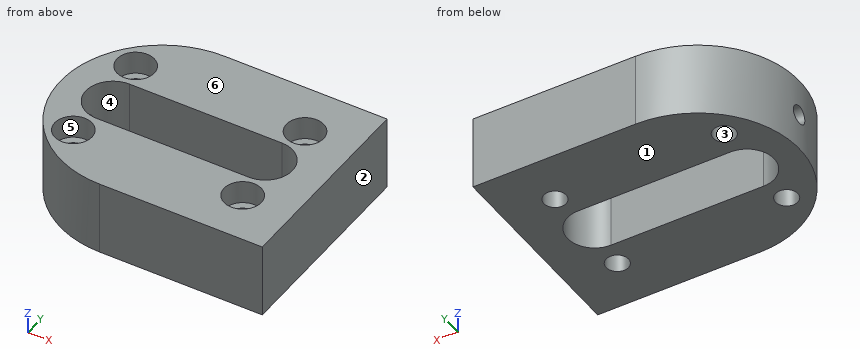
```python
from build123d import *

# Parameters (mm, degrees)
EXTRUDE_1_DEPTH           = 22
HOLE_WIZARD_1_D           = 6.6
HOLE_WIZARD_1_CBORE_D     = 11
HOLE_WIZARD_1_CBORE_DEPTH = 6.8
MM_1_REACH                = 86.291
MM_1_BORE_R               = 2.75


with BuildPart() as part:
    # 草图1 → 凸台-拉伸1 (new body)
    with BuildSketch(Plane.XY):
        with BuildLine():
            Line((-8, 30), (40, 30))
            Line((40, 30), (40, -30))
            Line((40, -30), (-8, -30))
            ThreePointArc((-8, -30), (-38, 0), (-8, 30))
        make_face()
        with BuildLine():
            Line((-22.5, 8), (22.5, 8))
            ThreePointArc((22.5, 8), (30.5, 0), (22.5, -8))
            Line((22.5, -8), (-22.5, -8))
            ThreePointArc((-22.5, -8), (-30.5, 0), (-22.5, 8))
        make_face(mode=Mode.SUBTRACT)
    extrude(amount=EXTRUDE_1_DEPTH)

    # 打孔尺寸(%根据)内六角圆柱头螺钉的类型1 (through all)
    with Locations(Plane(origin=(-25, 15, 22), x_dir=(1, 0, 0), z_dir=(0, 0, 1))):
        with Locations((0, 0), (0, -30), (50, 0), (50, -30)):
            CounterBoreHole(HOLE_WIZARD_1_D / 2, HOLE_WIZARD_1_CBORE_D / 2, HOLE_WIZARD_1_CBORE_DEPTH)

    # 大小mm 暗销孔1 bore (on position points) → 大小mm 暗销孔1 (cut, up to next)
    with BuildSketch(Plane(origin=(-38, 0, 11), x_dir=(0, 0, -1), z_dir=(-1, 0, 0)), mode=Mode.PRIVATE) as mm_1_sk1:
        Circle(MM_1_BORE_R)
    mm_1_tool1 = extrude(mm_1_sk1.sketch, amount=-MM_1_REACH, mode=Mode.PRIVATE) & part.part
    add(mm_1_tool1.solids().sort_by_distance((-38, 0, 11))[0], mode=Mode.SUBTRACT)


solid = part.part
```
Source: CAD feature listing. Evaluate the final solid. Frame: model axes, mm. Face numbers are marked on the shaded views. A direction names the side the tool comes from. Coordinates: 2 decimals unless noted, no trailing zeros. Loops run counter-clockwise (first coordinate to the right, second up) from the corner with the lowest first, then second, coordinate; pieces in that order, holes last. Notation, with made-up numbers: M 5.25,8 L 20.25,8 A25 cw 20.25,47 Z; hole C -31,72 d1. An arc over 180 degrees is marked long. Use a Markdown table: item, result. Add a question column.
Q1. Section query C-C, the plane y = 0. Return loops of the section in (x, z), and give its area (3 significant figures).
Q2. Draft query along X for the marked faces 1, 2 and 3. Return one class per face: pulls with the +X half, pulls with the -X half, needs draft (parallel to the pull), parting line crosses it, or undercut.
Q3. Access query for the marked faces 4, 5 and 6. Directions: +Z, -Z, +X, -X, +Y, -Y. A direction counts if a zero-diameter tool reaches every point of the face in a straight line with its end or side. Return the directions, or none.
Q4. Section query B-B, the plane z = 6.75. Return loops of the section in (x, y).
Q5. Section query A-A, the plane x = -5.5. Return loops of the section in (y, z).
Q6. Section query D-D, the plane x = -25. Return loops of the section in (y, z), and give its area (3 significant figures).
Q7. Material intervals for L1, parallel to Y at x = -23.5, z = 15.25; L2, parallel to Y at x = 0.5, z = 5; L3, parallel to X at y = -12, z = 14.75, sorted ascending.
Q8. First-contact query: pin 1 (5.5 mm diameter, centred on x = 25, y = 15, fed in from -Z); pin 2 (1 mm diameter, centred on x = -23, z = 14, fed in from -Y); pin 3 (9 mm diameter, centred on x = -25, y = 15, fed in from +Z). Flat tips, straight axial feed; report the tip coordinate or a pass-through.
Result:
| question | item | result |
|---|---|---|
| 1 | outline | M -38,0 L -30.5,0 L -30.5,8.25 L -38,8.25 Z; M -38,13.75 L -30.5,13.75 L -30.5,22 L -38,22 Z; M 30.5,0 L 40,0 L 40,22 L 30.5,22 Z |
| 1 | area | 333 mm2 |
| 2 | face 1 | needs draft |
| 2 | face 2 | pulls with the +X half |
| 2 | face 3 | undercut |
| 3 | face 4 | +Z, -Z |
| 3 | face 5 | +Z |
| 3 | face 6 | +Z, +X, -X, +Y, -Y |
| 4 | outline | M -8,-30 L 40,-30 L 40,30 L -8,30 A30 ccw Z; hole C -25,-15 d6.6; hole C -25,15 d6.6; hole M -22.5,-8 L 22.5,-8 A8 ccw 22.5,8 L -22.5,8 A8 ccw Z; hole C 25,-15 d6.6; hole C 25,15 d6.6 |
| 5 | outline | M -30,0 L -8,0 L -8,22 L -30,22 Z; M 8,0 L 30,0 L 30,22 L 8,22 Z |
| 6 | outline | M -24.72,0 L -18.3,0 L -18.3,15.2 L -20.5,15.2 L -20.5,22 L -24.72,22 Z; M -11.7,0 L -7.6,0 L -7.6,22 L -9.5,22 L -9.5,15.2 L -11.7,15.2 Z; M 7.6,0 L 11.7,0 L 11.7,15.2 L 9.5,15.2 L 9.5,22 L 7.6,22 Z; M 18.3,0 L 24.72,0 L 24.72,22 L 20.5,22 L 20.5,15.2 L 18.3,15.2 Z |
| 6 | area | 403 mm2 |
| 7 | L1 | y = -25.69 to -20.29, -9.71 to -7.94, 7.94 to 9.71, 20.29 to 25.69 |
| 7 | L2 | y = -30 to -8, 8 to 30 |
| 7 | L3 | x = -35.5 to -26.37, -23.63 to 23.63, 26.37 to 40 |
| 8 | pin 1 | passes through |
| 8 | pin 2 | stops at y = -26.26 |
| 8 | pin 3 | stops at z = 15.2 |
